```python
from build123d import *

# Parameters (mm, degrees)
SKETCH3_R               = 15.55
SKETCH3_R_2             = 8.15
BOSS_EXTRUDE4_DEPTH     = 6.5
SKETCH2_R               = 15.55
SKETCH2_R_2             = 8.15
BOSS_EXTRUDE5_DEPTH     = 6.5
CUT_EXTRUDE1_DEPTH      = 38.8
SKETCH5_R               = 1.6
CUT_EXTRUDE2_DEPTH      = 45.598710744
BOSS_EXTRUDE6_DEPTH     = 6.5
SKETCH9_W               = 6.5
SKETCH9_H               = 21.954006421
BOSS_EXTRUDE7_DEPTH     = 4
BOSS_EXTRUDE8_DEPTH     = 6.5
SKETCH12_W              = 6.5
SKETCH12_H              = 21.954006421
BOSS_EXTRUDE9_DEPTH     = 4
FILLET1_R               = 2
FILLET2_R               = 2
CUT_EXTRUDE3_DEPTH      = 50.233423685
SKETCH13_W              = 19.5
SKETCH13_H              = 7.8
BOSS_EXTRUDE10_DEPTH    = 38.8
FILLET3_R               = 2
SKETCH14_W              = 19.5
SKETCH14_H              = 5
BOSS_EXTRUDE11_DEPTH    = 6
SKETCH15_R              = 1.6
CUT_EXTRUDE4_DEPTH      = 65.138073781
SKETCH16_W              = 19.5
SKETCH16_H              = 5
BOSS_EXTRUDE12_DEPTH    = 6
SKETCH17_R              = 1.6
CUT_EXTRUDE5_DEPTH      = 65.138073781
SKETCH19_R              = 2.35
CUT_EXTRUDE7_DEPTH      = 10
FILLET4_R               = 1
SKETCH20_R              = 1.6
CUT_EXTRUDE8_DEPTH      = 57.651532835
CUT_EXTRUDE8_DEPTH_BACK = 57.651532835
FILLET5_R               = 1


with BuildPart() as part:
    # Sketch3 → Boss-Extrude4 (new body)
    with BuildSketch(Plane(origin=(0, 0, 0), x_dir=(0, 0, -1), z_dir=(1, 0, 0))):
        with Locations(Location((0, 0, 0), (0, 0, 180))):
            Circle(SKETCH3_R)
        with Locations(Location((0, 0, 0), (0, 0, 180))):
            Circle(SKETCH3_R_2, mode=Mode.SUBTRACT)
    extrude(amount=BOSS_EXTRUDE4_DEPTH)


with BuildPart() as body_2:
    # Sketch2 → Boss-Extrude5 (new body)
    with BuildSketch(Plane(origin=(32.3, 0, 0), x_dir=(0, 0, -1), z_dir=(1, 0, 0))):
        with Locations(Location((0, 0, 0), (0, 0, 180))):
            Circle(SKETCH2_R)
        with Locations(Location((0, 0, 0), (0, 0, 180))):
            Circle(SKETCH2_R_2, mode=Mode.SUBTRACT)
    extrude(amount=BOSS_EXTRUDE5_DEPTH)


with BuildPart() as cut_extrude1_tool:
    # Sketch4 → Cut-Extrude1 (new body)
    with BuildSketch(Plane(origin=(0, 0, 0), x_dir=(0, 0, -1), z_dir=(1, 0, 0))):
        with BuildLine():
            Line((0, 15.55), (0, -15.55))
            ThreePointArc((0, -15.55), (15.55, 0), (0, 15.55))
        make_face()
    extrude(amount=CUT_EXTRUDE1_DEPTH)


with BuildPart() as part_1:
    add(part.part)

    # Cut-Extrude1: cut by cut_extrude1_tool
    add(cut_extrude1_tool.part, mode=Mode.SUBTRACT)


with BuildPart() as body_2_1:
    add(body_2.part)

    # Cut-Extrude1: cut by cut_extrude1_tool
    add(cut_extrude1_tool.part, mode=Mode.SUBTRACT)


with BuildPart() as cut_extrude2_tool:
    # Sketch5 → Cut-Extrude2 (new, through all)
    with BuildSketch(Plane(origin=(0, 0, 0), x_dir=(-1, 0, 0), z_dir=(0, 0, -1))):
        with Locations((-35.55, 11.85)):
            Circle(SKETCH5_R)
        with Locations((-3.25, 11.85)):
            Circle(SKETCH5_R)
    extrude(amount=-CUT_EXTRUDE2_DEPTH)


with BuildPart() as part_2:
    add(part_1.part)

    # Cut-Extrude2: cut by cut_extrude2_tool
    add(cut_extrude2_tool.part, mode=Mode.SUBTRACT)

    # Sketch11 → Boss-Extrude8 (add)
    with BuildSketch(Plane.ZY):
        with BuildLine():
            ThreePointArc((15.5, -1.245993579), (10.545788255, -11.427547859), (0, -15.55))
            Line((0, -15.55), (0, -23.2))
            Line((0, -23.2), (15.5, -23.2))
            Line((15.5, -23.2), (15.5, -1.245993579))
        make_face()
    extrude(amount=-BOSS_EXTRUDE8_DEPTH)

    # Sketch12 → Boss-Extrude9 (add)
    with BuildSketch(Plane.XY.offset(15.5)):
        with Locations((3.25, -12.22299679)):
            Rectangle(SKETCH12_W, SKETCH12_H)
    extrude(amount=BOSS_EXTRUDE9_DEPTH)

    # Fillet2
    fillet2_edges = [part_2.edges().sort_by_distance(p)[0] for p in [
        (3.25, -1.245993579, 15.5),
    ]]
    fillet(fillet2_edges, radius=FILLET2_R)


with BuildPart() as body_2_2:
    add(body_2_1.part)

    # Cut-Extrude2: cut by cut_extrude2_tool
    add(cut_extrude2_tool.part, mode=Mode.SUBTRACT)

    # Sketch8 → Boss-Extrude6 (add)
    with BuildSketch(Plane(origin=(38.8, 0, 0), x_dir=(0, 0, -1), z_dir=(1, 0, 0))):
        with BuildLine():
            ThreePointArc((0, -19.2), (-8.691551143, -17.120074145), (-15.5, -11.330931118))
            Line((-15.5, -11.330931118), (-15.5, -23.2))
            Line((-15.5, -23.2), (0, -23.2))
            Line((0, -23.2), (0, -19.2))
        make_face()
        with BuildLine():
            ThreePointArc((0, -15.55), (-10.545788255, -11.427547859), (-15.5, -1.245993579))
            Line((-15.5, -1.245993579), (-15.5, -11.330931118))
            ThreePointArc((-15.5, -11.330931118), (-8.691551143, -17.120074145), (0, -19.2))
            Line((0, -19.2), (0, -15.55))
        make_face()
    extrude(amount=-BOSS_EXTRUDE6_DEPTH)

    # Sketch9 → Boss-Extrude7 (add)
    with BuildSketch(Plane.XY.offset(15.5)):
        with Locations((35.55, -12.22299679)):
            Rectangle(SKETCH9_W, SKETCH9_H)
    extrude(amount=BOSS_EXTRUDE7_DEPTH)

    # Fillet1
    fillet1_edges = [body_2_2.edges().sort_by_distance(p)[0] for p in [
        (35.55, -1.245993579, 15.5),
    ]]
    fillet(fillet1_edges, radius=FILLET1_R)


with BuildPart() as cut_extrude3_tool:
    # Sketch10 → Cut-Extrude3 (new, through all)
    with BuildSketch(Plane(origin=(38.8, 0, 0), x_dir=(0, 0, -1), z_dir=(1, 0, 0))):
        with BuildLine():
            Line((-19.5, -3.212198374), (-19.5, -1.245993579))
            Line((-19.5, -1.245993579), (-17.533795206, -1.245993579))
            ThreePointArc((-17.533795206, -1.245993579), (-18.924111949, -1.82188163), (-19.5, -3.212198374))
        make_face()
    extrude(amount=-CUT_EXTRUDE3_DEPTH)


with BuildPart() as part_3:
    add(part_2.part)

    # Cut-Extrude3: cut by cut_extrude3_tool
    add(cut_extrude3_tool.part, mode=Mode.SUBTRACT)



with BuildPart() as body_2_3:
    add(body_2_2.part)

    # Cut-Extrude3: cut by cut_extrude3_tool
    add(cut_extrude3_tool.part, mode=Mode.SUBTRACT)


with BuildPart() as part_4:
    add(part_3.part)

    add(body_2_3.part)  # Boss-Extrude10 merges body 2
    # Sketch13 → Boss-Extrude10 (add)
    with BuildSketch(Plane(origin=(38.8, 0, 0), x_dir=(0, 0, -1), z_dir=(1, 0, 0))):
        with Locations((-9.75, -27.1)):
            Rectangle(SKETCH13_W, SKETCH13_H)
    extrude(amount=-BOSS_EXTRUDE10_DEPTH)

    # Fillet3
    fillet3_edges = [part_4.edges().sort_by_distance(p)[0] for p in [
        (6.5, -23.2, 9.75),
        (32.3, -23.2, 9.75),
    ]]
    fillet(fillet3_edges, radius=FILLET3_R)

    # Sketch14 → Boss-Extrude11 (add)
    with BuildSketch(Plane(origin=(38.8, 0, 0), x_dir=(0, 0, -1), z_dir=(1, 0, 0))):
        with Locations((-9.75, -28.5)):
            Rectangle(SKETCH14_W, SKETCH14_H)
    extrude(amount=BOSS_EXTRUDE11_DEPTH)

    # Sketch15 → Cut-Extrude4 (cut, through all)
    with BuildSketch(Plane(origin=(0, -26, 0), x_dir=(1, 0, 0), z_dir=(0, 1, 0))):
        with Locations(Location((41.8, -9.75, 0), (0, 0, 270))):
            Circle(SKETCH15_R)
    extrude(amount=-CUT_EXTRUDE4_DEPTH, mode=Mode.SUBTRACT)

    # Sketch16 → Boss-Extrude12 (add)
    with BuildSketch(Plane.ZY):
        with Locations((9.75, -28.5)):
            Rectangle(SKETCH16_W, SKETCH16_H)
    extrude(amount=BOSS_EXTRUDE12_DEPTH)

    # Sketch17 → Cut-Extrude5 (cut, through all)
    with BuildSketch(Plane(origin=(0, -26, 0), x_dir=(1, 0, 0), z_dir=(0, 1, 0))):
        with Locations(Location((-3, -9.75, 0), (0, 0, 270))):
            Circle(SKETCH17_R)
    extrude(amount=-CUT_EXTRUDE5_DEPTH, mode=Mode.SUBTRACT)

    # Sketch19 → Cut-Extrude7 (cut)
    with BuildSketch(Plane(origin=(0, 0, 0), x_dir=(-1, 0, 0), z_dir=(0, 0, -1))):
        with Locations((-8.5, -27.1)):
            Circle(SKETCH19_R)
        with Locations((-30.3, -27.1)):
            Circle(SKETCH19_R)
    extrude(amount=-CUT_EXTRUDE7_DEPTH, mode=Mode.SUBTRACT)

    # Fillet4
    fillet4_edges = [part_4.edges().sort_by_distance(p)[0] for p in [
        (6.5, -0.690267327, 16.150294811),
        (6.5, -1.82188163, 18.924111949),
        (6.5, 11.229228387, 10.756715569),
        (0, -0.690267327, 16.150294811),
        (0, 11.229228387, 10.756715569),
        (0, -1.82188163, 18.924111949),
        (19.4, -23.2, 19.5),
        (6.5, -12.206099187, 19.5),
        (31.714213562, -22.614213562, 19.5),
        (7.085786438, -22.614213562, 19.5),
        (38.8, -14.606099187, 19.5),
        (0, -14.606099187, 19.5),
        (32.3, 11.229228387, 10.756715569),
        (38.8, 11.229228387, 10.756715569),
        (38.8, -0.690267327, 16.150294811),
        (32.3, -0.690267327, 16.150294811),
        (32.3, -12.206099187, 19.5),
        (38.8, -1.82188163, 18.924111949),
        (32.3, -1.82188163, 18.924111949),
    ]]
    fillet(fillet4_edges, radius=FILLET4_R)

    # Sketch20 → Cut-Extrude8 (cut, two sides)
    with BuildSketch(Plane.XY.offset(15.535641906)) as cut_extrude8_sk:
        with Locations((3.25, 0)):
            Circle(SKETCH20_R)
        with Locations((35.55, 0)):
            Circle(SKETCH20_R)
    extrude(amount=CUT_EXTRUDE8_DEPTH, mode=Mode.SUBTRACT)
    extrude(cut_extrude8_sk.sketch, amount=-CUT_EXTRUDE8_DEPTH_BACK, mode=Mode.SUBTRACT)

    # Fillet5
    fillet5_edges = [part_4.edges().sort_by_distance(p)[0] for p in [
        (44.8, -28.5, 19.5),
        (41.3, -26, 19.5),
        (19.4, -31, 19.5),
        (-6, -28.5, 19.5),
        (-2.5, -26, 19.5),
    ]]
    fillet(fillet5_edges, radius=FILLET5_R)


solid = part_4.part
```
Geometry check sheet. Reference: the model listing, model coordinates, mm. A direction names the side the tool comes from. Coordinates: 2 decimals unless noted, no trailing zeros. Order: outer loops, then holes, each group sorted by start corner. A loop starts at its lowest first (then second) coordinate and runs counter-clockwise, first axis right, second up. Notation, with made-up numbers: M 11.5,79.5 L 26.5,79.5 A26 cw 26.5,117.5 Z; hole C 47.25,-37.75 d7. An arc over 180 degrees is marked long. One line per question, with ' | ' between items. Start each with the question number.
Item 1: Material ranges on L1, parallel to X at y = 11.85, z = 6.5; L2, parallel to X at y = -13, z = 17.5; L3, parallel to Y at x = 8.5, z = 6.25, recorded low to high. Write a range as [from, to].
Item 2: Cross-section at A-A on y = -12.5. Enter the section's corners in (x, z).
Item 3: Cross-section at B-B on x = 41.8. Enter the section's corners in (y, z), then the cut area to 3 significant figures.
Item 4: Set-up check for faces 1 (the flat face through (6.5, -8, 9)), 2 (the flat face through (20, -26, 19.5)), 3 (the flat face through (30, -27, 10)), 4 (the flat face through (44.8, -28, 9)), 5 (the flat face through (-3, -26, 7)): record each of +Z, -Z, +X, -X, +Y, -Y from which the full face is reachable in a straight line by a thin tool's end or side.
Item 5: Draft check along X on faces 6 (the flat face through (32.3, -8, 9)), 7 (the flat face through (20, -25, 0)), 8 (the flat face through (38.8, -10, 9)), 9 (the flat face through (20, -23.2, 9)). Enter one of: pulls with the +X half, pulls with the -X half, needs draft (parallel to the pull), parting line crosses it, or undercut.
Item 6: Gauge pin test, flat ends, axial feed: pin 1 (6 mm diameter, centred on x = 16.5, z = 8, fed in from +Y); pin 2 (2.5 mm diameter, centred on x = 8, y = -26.5, fed in from -Z); pin 3 (5.5 mm diameter, centred on y = -15, z = 10.5, fed in from -X). Record the tip position at first contact, or that the pin passes through.
Item 7: Cross-section at D-D on x = 13. Enter the section's corners in (y, z).
Item 8: Cross-section at C-C on x = 35.55. Enter the section's corners in (y, z), then the cut area to 3 significant figures.
Findings:
1) L1: x = [0, 1.65], [4.85, 6.5], [32.3, 33.95], [37.15, 38.8] | L2: x = [0, 6.5], [32.3, 38.8] | L3: y = [-31, -29.45], [-24.75, -23.2]
2) outline: M 0,0 L 6.5,0 L 6.5,18.5 A1 ccw 5.5,19.5 L 1,19.5 A1 ccw 0,18.5 Z; M 32.3,0 L 38.8,0 L 38.8,18.5 A1 ccw 37.8,19.5 L 33.3,19.5 A1 ccw 32.3,18.5 Z
3) outline: M -31,0 L -26,0 L -26,8.15 L -31,8.15 Z; M -31,11.35 L -26,11.35 L -26,18.5 A1 ccw -27,19.5 L -30,19.5 A1 ccw -31,18.5 Z | area: 81.1 mm²
4) face 1: +Z, -Z, +Y | face 2: +Z, +X, -X, +Y, -Y | face 3: -Z | face 4: +Z, -Z, +X, +Y, -Y | face 5: +Z, -Z, -X, +Y
5) face 6: undercut | face 7: needs draft | face 8: pulls with the +X half | face 9: undercut
6) pin 1: stops at y = -23.2 | pin 2: stops at z = 10 | pin 3: stops at x = 0
7) outline: M -31,0 L -23.2,0 L -23.2,18.5 A1 ccw -24.2,19.5 L -30,19.5 A1 ccw -31,18.5 Z
8) outline: M -31,0 L -8.15,0 A8.15 cw -1.6,7.99 L -1.6,18.66 A1.97 ccw -3.21,19.5 L -30,19.5 A1 ccw -31,18.5 Z; M 1.6,7.99 A8.15 cw 8.15,0 L 10.25,0 L 10.25,11.69 A15.55 ccw 1.6,15.47 Z; M 13.45,0 L 15.55,0 A15.55 ccw 13.45,7.8 Z | area: 627 mm²
